Model file for the job. Use its own axes, mm. A direction names the side the tool comes from. Round coordinates to 2 decimals unless told otherwise and drop trailing zeros. Loops run counter-clockwise (first coordinate to the right, second up) from the corner with the lowest first, then second, coordinate; pieces in that order, holes last. Notation, with made-up numbers: M -34,81.5 L 17,81.5 A36 ccw 17,120.5 Z; hole C -29,14 d6. An arc over 180 degrees is marked long. Answer in a Markdown table with one row per item.
Autodesk Inventor part; units mm, degrees
ref_plane "YZ Plane" through (0, 0, 0) normal (1, 0, 0) x (0, 1, 0)
ref_plane "XZ Plane" through (0, 0, 0) normal (0, 1, 0) x (-1, 0, 0)
ref_plane "XY Plane" through (0, 0, 0) normal (0, 0, 1) x (1, 0, 0)
sketch "Skizze1" plane through (0, 0, 0) normal (0, 0, 1) x (1, 0, 0)
  circle A0 centre (0, 0) radius 80.1 construction
  circle A1 centre (0, 0) radius 93.8 construction
  circle A2 centre (0, 0) radius 80.6
  circle A3 centre (0, 0) radius 91.8
  arc A4 (5.5, 85.9242) -> (-5.5, 85.9242) centre (0, 0) ccw
  line L0 (-5.5, 85.9242) -> (-5.5, 80.4121)
  line L1 (5.5, 85.9242) -> (5.5, 80.4121)
  point P0 (0, 86.1)
  dimension "d0" = 187.6
  dimension "d1" = 160.2
  dimension "d2" = 2
  dimension "d3" = 0.5
  dimension "d6" = 6
  dimension "d7" = 11
extrude "Extrusion1" add sketch "Skizze1" along normal blind 5
sketch "Skizze2" plane through (0, 0, 5) normal (0, 0, 1) x (1, 0, 0)
  circle A0 centre (-86.2, 0) radius 2.6
  circle A1 centre (86.2, 0) radius 2.6
  line L0 (-86.2, 0) -> (86.2, 0) construction
  arc A2 (-5.5, 80.4121) -> (5.5, 80.4121) centre (0, 0) ccw construction
  point P0 (-80.6, 0)
  point P1 (80.6, 0)
  dimension "d8" = 5.2
  dimension "d9" = 5.6
  dimension "d10" = 5.6
extrude "Extrusion2" cut sketch "Skizze2" against normal blind 5
properties part number "Montage_Ring_Vorne"
1. Pin check, flat tips, straight feed: pin 1 (3 mm diameter, centred on x = 64.5, z = 1, fed in from -Y); pin 2 (1.5 mm diameter, centred on y = 84, z = 3.5, fed in from -X); pin 3 (3 mm diameter, centred on x = -16, z = 3, fed in from -Y). Stop position of each tip, or through.
Verdict:
| item | result |
|---|---|
| pin 1 | stops at y = -66.77 |
| pin 2 | stops at x = -38.69 |
| pin 3 | stops at y = -90.65 |
2. Mould opens along Y. For faces 3 (the cylindrical face through (-83.72, 0.78, 2.54)), 4 (the cylindrical face through (87.561, -27.574, 2.465)), 5 (the flat face through (0, -81, 5)) say: +Y half, -Y half, draft (parallel to the pull), parting line (faces both ways), or undercut.
Verdict:
| item | result |
|---|---|
| face 3 | undercut |
| face 4 | parting line |
| face 5 | draft |
3. Tool access for faces 1 (the cylindrical face through (-0.1, 86.1, 2.5)), 2 (the flat face through (0, -81, 0)): list every direction of +Z, -Z, +X, -X, +Y, -Y with a clear straight run to the whole face (end or side of a thin tool).
Verdict:
| item | result |
|---|---|
| face 1 | +Z, -Z |
| face 2 | -Z, +X, -X, +Y, -Y |
4. Saw through at C-C (z = 3.35). Write the cut outline in (x, y), and give its area (3 significant figures).
Verdict:
| item | result |
|---|---|
| outline | C 0,0 d183.6; hole C -86.2,0 d5.2; hole M -5.5,80.41 A80.6 ccw long 5.5,80.41 L 5.5,85.92 A86.1 ccw -5.5,85.92 Z; hole C 86.2,0 d5.2 |
| area | 5,960 mm² |
5. Wall check: probe 1 along Y at (x, z) = (72.5, 1.65); probe 2 along Y at (x, z) = (54, 4.4); probe 3 along X at (y, z) = (18.5, 3.05). Give the ranges that are in metal, low to high.
Verdict:
| item | result |
|---|---|
| probe 1 | y = -56.31 to -35.22, 35.22 to 56.31 |
| probe 2 | y = -74.24 to -59.84, 59.84 to 74.24 |
| probe 3 | x = -89.92 to -78.45, 78.45 to 89.92 |
6. Saw through at B-B (y = -42). Write the cut outline in (x, z).
Verdict:
| item | result |
|---|---|
| outline | M -81.63,0 L -68.79,0 L -68.79,5 L -81.63,5 Z; M 68.79,0 L 81.63,0 L 81.63,5 L 68.79,5 Z |
7. Saw through at A-A (x = 0). Write the cut outline in (y, z), and give its area (3 significant figures).
Verdict:
| item | result |
|---|---|
| outline | M -91.8,0 L -80.6,0 L -80.6,5 L -91.8,5 Z; M 86.1,0 L 91.8,0 L 91.8,5 L 86.1,5 Z |
| area | 84.5 mm² |
